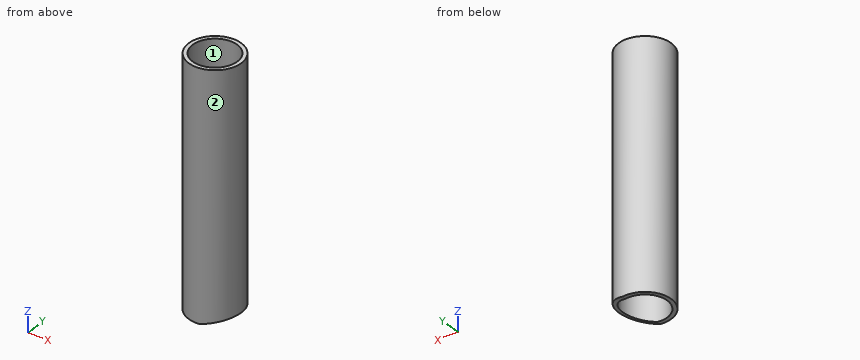
Autodesk Inventor part; units mm, degrees
ref_plane "Start Plane" through (0, 0, -24.13) normal (0, 0, 1) x (1, 0, 0)
ref_plane "End Plane" through (0, 0, 200) normal (0, 0, 1) x (1, 0, 0)
ref_plane "Work Plane4" through (-1133.3597, 0, -328.664) normal (0.2588, 0, -0.9659) x (-0.9659, 0, -0.2588)
ref_plane "Start Plane" through (0, 0, -24.13) normal (0, 0, 1) x (1, 0, 0)
ref_plane "End Plane" through (0, 0, 200) normal (0, 0, 1) x (1, 0, 0)
sketch "Sketch" plane through (0, 0, 0) normal (0, 0, 1) x (1, 0, 0)
  circle A0 centre (0, 0) radius 20.447
  circle A1 centre (0, 0) radius 24.13
  dimension "d0" = 48.26
  dimension "d1" = 3.683
extrude "Body" add sketch "Sketch" along normal up to surface (224.13 mm away) from surface at -24.13
sketch "Sketch3" plane through (0, 0, 0) normal (0, 0, 1) x (1, 0, 0)
  line L0 (0, 0) -> (10, 0)
ref_plane "Work Plane3" through (0, 0, 0) normal (0, -1, 0) x (1, 0, 0)
ref_plane "Work Plane4" through (-1133.3597, 0, -328.664) normal (0.2588, 0, -0.9659) x (-0.9659, 0, -0.2588)
split "Split1" plane through (-1133.3597, 0, -328.664) removes the side toward (0.2588, 0, -0.9659)
ref_plane "Work Plane5" through (0, 2000, -24.13) normal (0, 0, -1) x (-1, 0, 0)
split "Split2" plane through (0, 2000, -24.13) removes the side toward (0, 0, -1)
sketch "Sketch4" plane through (0, 0, 0) normal (0, -1, 0) x (1, 0, 0)
  line L0 (-2, -24.13) -> (12, -24.13)
  line L1 (-2, 200) -> (12, 200)
  dimension "d7" = 224.13
equation "\"d0\" = G_H"
equation "\"d1\" = G_T"
equation "\"d2\" = G_L"
equation "\"G_H\" = 48.26"
equation "\"G_T\" = 3.683"
equation "\"G_L\" = d7"
equation "\"G_OFFSET_START\" = 24.13"
equation "\"G_OFFSET_END\" = 0"
equation "\"d4\" = -G_OFFSET_START"
equation "\"d5\" = G_OFFSET_END + B_L"
equation "\"B_L\" = 200"
properties part number "ANSI - 1 1/2 x 0.145 - 8.824" material "Steel, Mild"
Part model, mm, in its own coordinate system. Face numbers are marked on the shaded views. Coordinates: 2 decimals unless noted, no trailing zeros. Order: outer loops, then holes, each group sorted by start corner. A loop starts at its lowest first (then second) coordinate and runs counter-clockwise, first axis right, second up. Notation, with made-up numbers: (16.5, 81.5) - (33.5, 81.5) arc R14 cw to (33.5, 105.5) - close; hole circle Ø11 at (-15.5, -3.5). An arc over 180 degrees is marked (long way). Use CSV: the item, a comma, the result in double quotes.
Item 1: Saw through at A-A on x = 0. Give the cut face in (y, z).
Solved:
outline,"(-24.13, -24.13) - (-20.45, -24.13) - (-20.45, 200) - (-24.13, 200) - close; (20.45, -24.13) - (24.13, -24.13) - (24.13, 200) - (20.45, 200) - close"
Item 2: Drop flat-ended pins along their axis: P1, Ø12, axis at x = 4.5, z = 162.5, coming from the +Y side; P2, Ø4, axis at y = 10.5, z = 115, coming from the +X side; P3, Ø3, axis at x = 11, z = 40.5, coming from the -Y side. Give the stop position or say it passes through.
Solved:
P1,"stops at y = 24.13"
P2,"stops at x = 22.58"
P3,"stops at y = -22.18"
Item 3: Saw through at B-B on y = 0. Give the cut face in (x, z).
Solved:
outline,"(-24.13, -24.13) - (-20.45, -24.13) - (-20.45, 200) - (-24.13, 200) - close; (20.45, -19.5) - (24.13, -18.52) - (24.13, 200) - (20.45, 200) - close"
Item 4: Saw through at C-C on z = 52.5. Give the cut face in (x, y).
Solved:
outline,"circle Ø48.26 at (0, 0); hole circle Ø40.89 at (0, 0)"
Item 5: Probe probe 1 along Y at (x, z) = (0, 134); probe 2 along X at (y, z) = (-0.5, 162); probe 3 along Y at (x, z) = (5.5, 157). List the from-to ranges inside material, lowest first.
Solved:
probe 1,"y = -24.13 to -20.45, 20.45 to 24.13"
probe 2,"x = -24.12 to -20.44, 20.44 to 24.12"
probe 3,"y = -23.49 to -19.69, 19.69 to 23.49"
Item 6: Mould opens along Y. For the marked faces 1 and 2 say: +Y half, -Y half, draft (parallel to the pull), parting line (faces both ways), or undercut.
Solved:
face 1,"undercut"
face 2,"parting line"
